Here's how the part is built. I have some questions about the finished solid (model axes, mm). Face numbers are marked on the shaded views. Coordinates: 2 decimals unless noted, no trailing zeros. Write each loop counter-clockwise with the first axis right and the second up, starting at its lowest first coordinate (ties: lowest second). Pieces come first, ordered by that corner, then holes. Notation, with made-up numbers: (77.5, 17.25) -> (88.5, 17.25) arc R22 cw to (88.5, 47.25) -> close; hole circle Ø8 at (-34, -6). An arc over 180 degrees is marked (long way). Use CSV: the item, a comma, the result in double quotes. Start each with the question number.
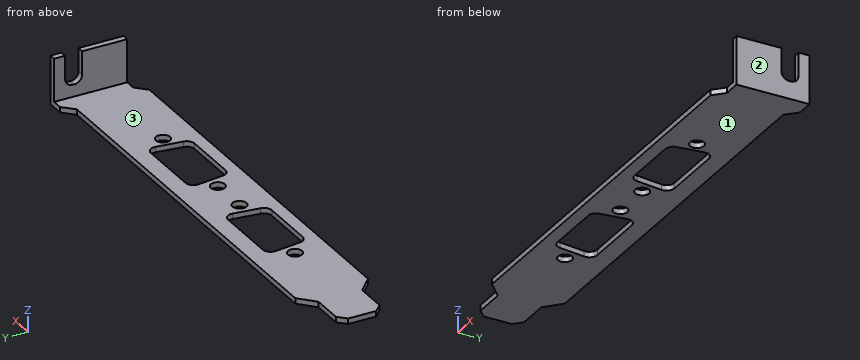
Autodesk Fusion 360 part; units mm, degrees
sketch "스케치1" plane through (0, 0, 0) normal (0, 0, 1) x (1, 0, 0)
  line L0 (14, 18.6) -> (114.5, 18.6)
  line L1 (114.5, 18.6) -> (114.5, 0)
  line L2 (114.5, 0) -> (14, 0)
  line L3 (14, 0) -> (14, 18.6)
  line L4 (0, 14.875) -> (10, 14.875)
  line L5 (10, 14.875) -> (10, 3.725)
  line L6 (10, 3.725) -> (0, 3.725)
  line L7 (0, 3.725) -> (0, 14.875)
  line L8 (0, 9.3) -> (10, 9.3) construction
  line L9 (10, 14.875) -> (14, 18.6)
  line L10 (10, 3.725) -> (14, 0)
  line L11 (1.75, 0) -> (22.5, 0)
  line L12 (0, 1.75) -> (0, 22.5)
  line L13 (120, 21.36) -> (117.25, 21.36)
  line L14 (117.25, 21.36) -> (117.25, 2.66)
  line L15 (117.25, 2.66) -> (120, 2.66)
  line L16 (120, 2.66) -> (120, 21.36)
  line L17 (114.5, 0) -> (144, 0) construction
  line L18 (114.5, 18.6) -> (117.25, 21.36)
  line L19 (114.5, 0) -> (117.25, 2.66)
  line L20 (120, 21.36) -> (121.7, 21.36)
  line L21 (121.7, 21.36) -> (121.7, 2.66)
  line L22 (121.7, 2.66) -> (120, 2.66)
  line L23 (120, 2.66) -> (120, 21.36)
  dimension "d1" = 100.5
  dimension "d2" = 18.6
  dimension "d3" = 10
  dimension "d4" = 11.15
  dimension "d5" = 4
  dimension "d6" = 18.7
  dimension "d7" = 2.66
  dimension "d8" = 2.75
  dimension "d9" = 2.75
  dimension "d10" = 1.7
extrude "돌출1" add sketch "스케치1" along normal blind 1.4 contours L0 L1 L2 L3 L11 | L3 L5 L9 L10 | L1 L14 L18 L19 | L4 L5 L6 L7 L12 | L13 L14 L15 L16 L23
extrude "돌출2" add sketch "스케치1" along normal blind 12.4 contours L16 L20 L21 L22 L23
chamfer "모따기1" distance 2 angle 45 2 edges at (0, 3.725, 0.7) (0, 14.875, 0.7)
sketch "스케치2" plane through (121.7, 0, 0) normal (1, 0, 0) x (0, 1, 0)
  line L0 (2.66, 0) -> (21.36, 0)
  line L1 (21.36, 0) -> (21.36, 12.4)
  line L2 (21.36, 12.4) -> (2.66, 12.4)
  line L3 (2.66, 12.4) -> (2.66, 0)
  line L4 (14.16, 12.4) -> (18.56, 12.4)
  line L5 (18.56, 12.4) -> (18.56, 4.5)
  line L6 (18.56, 4.5) -> (14.16, 4.5)
  line L7 (14.16, 4.5) -> (14.16, 12.4)
  dimension "d16" = 2.8
  dimension "d17" = 4.4
  dimension "d18" = 7.9
extrude "돌출3" cut sketch "스케치2" against normal blind 3 contours L2 L4 L5 L6 L7
fillet "모깎기1" radius 2 2 edges at (120.85, 14.16, 4.5) (120.85, 18.56, 4.5)
sketch "스케치3" plane through (0, 0, 1.4) normal (0, 0, 1) x (-1, 0, 0)
  line L0 (-2, -14.875) -> (0, -12.875)
  line L1 (0, -12.875) -> (0, -5.725)
  line L2 (0, -5.725) -> (-2, -3.725)
  line L3 (-2, -3.725) -> (-10, -3.725)
  line L4 (-10, -3.725) -> (-14, 0)
  line L5 (-14, 0) -> (-114.5, 0)
  line L6 (-114.5, 0) -> (-117.25, -2.66)
  line L7 (-117.25, -2.66) -> (-120, -2.66)
  line L8 (-120, -2.66) -> (-120, -21.36)
  line L9 (-120, -21.36) -> (-117.25, -21.36)
  line L10 (-117.25, -21.36) -> (-114.5, -18.6)
  line L11 (-114.5, -18.6) -> (-14, -18.6)
  line L12 (-14, -18.6) -> (-10, -14.875)
  line L13 (-10, -14.875) -> (-2, -14.875)
  line L14 (7.5, -3.3) -> (-137.5, -3.3) construction
  line L15 (-114.5, 0) -> (-14, 0)
  line L16 (7.5, -14) -> (-137.5, -14) construction
  line L17 (-70.5, -14) -> (-91, -14)
  line L18 (-71.9, -3.3) -> (-89.6, -3.3)
  line L19 (-70.5, -14) -> (-71.9, -3.3)
  line L20 (-91, -14) -> (-89.6, -3.3)
  line L21 (-80.75, -32) -> (-80.75, 14) construction
  line L22 (-70.5, -26) -> (-70.5, 12) construction
  line L23 (-91, -26) -> (-91, 12) construction
  circle A0 centre (-67.995, -8.4) radius 1.8
  circle A1 centre (-93.205, -8.4) radius 1.8
  line L24 (-91.405, -12) -> (-91.405, -5.5195) construction
  line L25 (-69.795, -12) -> (-69.795, -5.5195) construction
  line L26 (-66.5, -6.6) -> (-95, -6.6) construction
  line L27 (-35, -14) -> (-55.5, -14)
  line L28 (-36.4, -3.3) -> (-54.1, -3.3)
  line L29 (-35, -14) -> (-36.4, -3.3)
  line L30 (-55.5, -14) -> (-54.1, -3.3)
  circle A2 centre (-32.495, -8.4) radius 1.8
  circle A3 centre (-58.005, -8.4) radius 1.8
  line L31 (-35, -26) -> (-35, 12) construction
  line L32 (-55.5, -26) -> (-55.5, 12) construction
  line L33 (-34.295, -12) -> (-34.295, -5.5195) construction
  line L34 (-56.205, -12) -> (-56.205, -5.5195) construction
  dimension "d23" = 3.3
  dimension "d24" = 10.7
  dimension "d25" = 20.5
  dimension "d26" = 17.7
  dimension "d27" = 29
  dimension "d28" = 3.6
  dimension "d30" = 0.705
  dimension "d31" = 0.405
  dimension "d32" = 3.3
  dimension "d37" = 3.6
  dimension "d38" = 0.705
  dimension "d39" = 0.705
  dimension "d40" = 15
extrude "돌출4" cut sketch "스케치3" against normal blind 2 contours L17 L18 L19 L20 | A0 | A1
fillet "모깎기2" radius 2 4 edges at (91, 14, 0.7) (70.5, 14, 0.7) (89.6, 3.3, 0.7) (71.9, 3.3, 0.7)
extrude "돌출5" cut sketch "스케치3" against normal blind 4 contours L27 L28 L29 L30 | A2 | A3
fillet "모깎기3" radius 2 4 edges at (35, 14, 0.7) (55.5, 14, 0.7) (36.4, 3.3, 0.7) (54.1, 3.3, 0.7)
Item 1: I want a section at D-D on x = 27. Please give me the cut outline in (y, z), then the cut area to 3 significant figures.
Item 2: Thinking about a two-plate mould opening in Z: for the marked faces 1, 2 and 3, which applies, +Z half, -Z half, draft (parallel to the pull), parting line (faces both ways), or undercut?
Item 3: I want a section at C-C on y = 8.4. Count the separate pieces of the cut face and the enclosed holes in it, then the cut area to 3 significant figures.
Item 4: I want a section at B-B on z = 10.5. Please give me the cut outline in (x, y), then the cut area to 3 significant figures.
Item 5: If I drill on line 1 along X through (y, z) = (12.5, 1.25); line 2 along X through (y, z) = (5, 7.25); line 3 along Z through (x, y) = (18, 9.25), over which ranges is the centre line in solid material (lowest first)?
Item 6: I want a section at A-A on x = 39.5. Please give me the cut outline in (y, z), then the cut area to 3 significant figures.
Item 7: I'm going to push flat-ended pins straight in: pin 1 (6.5 mm diameter, centred on x = 55, y = 6, fed in from +Z); pin 2 (0.7 mm diameter, centred on x = 41.5, z = 1, fed in from +Y); pin 3 (5 mm diameter, centred on x = 119.5, z = 4, fed in from -Y); pin 4 (2 mm diameter, centred on x = 93.205, y = 8.4, fed in from -Z). Where does each tip first touch, or does it pass through?
Geometry says:
1,outline,"(0, 0) -> (18.6, 0) -> (18.6, 1.4) -> (0, 1.4) -> close"
1,area,"26.0 mm2"
2,face 1,"-Z half"
2,face 2,"draft"
2,face 3,"+Z half"
3,separate pieces,"7"
3,enclosed holes,"0"
3,area,"116 mm2"
4,outline,"(120, 2.66) -> (121.7, 2.66) -> (121.7, 14.16) -> (120, 14.16) -> close; (120, 18.56) -> (121.7, 18.56) -> (121.7, 21.36) -> (120, 21.36) -> close"
4,area,"24.3 mm2"
5,line 1,"0 to 35.34, 55.16 to 70.84, 90.66 to 121.7"
5,line 2,"120 to 121.7"
5,line 3,"0 to 1.4"
6,outline,"(0, 0) -> (3.3, 0) -> (3.3, 1.4) -> (0, 1.4) -> close; (14, 0) -> (18.6, 0) -> (18.6, 1.4) -> (14, 1.4) -> close"
6,area,"11.1 mm2"
7,pin 1,"z = 1.4"
7,pin 2,"y = 18.6"
7,pin 3,"y = 2.66"
7,pin 4,"through"
